Autodesk Inventor part; units mm, degrees
ref_plane "YZ Plane" through (0, 0, 0) normal (1, 0, 0) x (0, 1, 0)
ref_plane "XZ Plane" through (0, 0, 0) normal (0, 1, 0) x (-1, 0, 0)
ref_plane "XY Plane" through (0, 0, 0) normal (0, 0, 1) x (1, 0, 0)
sketch "スケッチ1" plane through (0, 0, 0) normal (0, 1, 0) x (-1, 0, 0)
  circle A0 centre (0, 0) radius 1.15
  circle A1 centre (0, 0) radius 2
  circle A2 centre (0, 0) radius 5
  line L0 (0, 0) -> (7, 0)
  line L1 (7, 0) -> (7, 4.5)
  line L2 (7, 4.5) -> (0, 4.5)
  line L3 (0, 4.5) -> (0, 0)
  line L4 (0, 0) -> (7, 0)
  line L5 (7, 0) -> (7, -5)
  line L6 (7, -5) -> (0, -5)
  line L7 (0, -5) -> (0, 0)
  line L8 (0, 4.5) -> (-2, 4.5)
  line L9 (-2, 4.5) -> (-2, 0)
  line L10 (-2, 0) -> (0, 0)
  line L11 (0, 0) -> (0, 4.5)
  circle A3 centre (0, 0) radius 3
  line L12 (-2, 0) -> (-2, -5)
  line L13 (-2, -5) -> (0, -5)
  line L14 (2, 0) -> (2, -5)
  circle A4 centre (0, 0) radius 4.9244
  line L15 (-2, 0) -> (-4.9244, 0)
  line L16 (0, -4.9244) -> (0, -5.9244)
  line L17 (0, -5.9244) -> (7, -5.9244)
  line L18 (7, -5.9244) -> (7, -5)
  line L19 (7, -5) -> (0, -5.9244)
  line L20 (0, -5.9244) -> (4.9138, -5)
  line L21 (0, -5) -> (0, -7)
  line L22 (0, -7) -> (4.9138, -5)
  point P0 (0, 2)
  point P1 (-2, 2.2361)
  point P2 (-2, -2.2361)
  point P3 (-2, -4.5826)
  point P4 (-2, -4.5)
  point P5 (0, -4.9244)
  dimension "d2" = 10
  dimension "d0" = 2.3
  dimension "d1" = 4
  dimension "d3" = 7
  dimension "d4" = 4.5
  dimension "d5" = 6
  dimension "d22" = 1
  dimension "d34" = 5
  dimension "d39" = 2
extrude "押し出し1" add sketch "スケッチ1" along normal blind 4.5 contours A1 L3 A3 L0 | L0 A3 L14 | A3 L3 L2 A4 L0 | L0 A4 L14 A3 | A4 L2 A2 L0 | L0 A2 L14 A4 | L0 L5 L6 L14 A2 | A2 L2 L1 L0
extrude "押し出し2" add sketch "スケッチ1" along normal blind 3 contours A1 L9 A3 L3 | L15 A3 L9 | L12 A3 L15 | A3 L9 L8 L3 | A3 L15 A4 L9 | L12 A4 L15 A3
extrude "押し出し3" add sketch "スケッチ1" against normal blind 1 contours L0 A1 L7 A0 | A0 L3 A1 L0 | A0 L10 A1 L3 | L7 A1 L10 A0 | L14 A3 L7 A1 | A1 L3 A3 L0 | L0 A3 L14 | A1 L9 A3 L3 | L7 A3 L12 A1 | A3 L3 L2 A4 L0 | L0 A4 L14 A3 | L14 A4 L7 A3 | L15 A3 L9 | L12 A3 L15 | A3 L9 L8 L3 | L7 A4 L12 A3 | A4 L2 A2 L0 | L0 A2 L14 A4 | L14 A2 L7 A4 | A3 L15 A4 L9 | L12 A4 L15 A3 | L0 L5 L6 L14 A2 | A2 L2 L1 L0 | L14 L6 A2 | L6 L20 L16 | L19 L22 L17 | L20 L22 L19 | L17 L22 L21
sketch "スケッチ2" plane through (0, 4.5, 0) normal (0, 1, 0) x (1, 0, 0)
  circle A0 centre (0, 0) radius 1.15
  circle A1 centre (0, 0) radius 2
  circle A2 centre (0, 0) radius 4.9244
  line L0 (0, 0) -> (2, 0)
  line L1 (2, 0) -> (2, -4.5)
  line L2 (2, -4.5) -> (0, -4.5)
  line L3 (0, -4.5) -> (0, 0)
  line L4 (-2, 5) -> (-7, 5)
  line L5 (0, -4.5) -> (-7, -4.5)
  line L6 (-7, -4.5) -> (-7, 5)
  line L7 (-7, 5) -> (0, 5)
  line L8 (0, 5) -> (0, -4.5)
  line L9 (0, 0) -> (2, 0)
  line L10 (2, 0) -> (2, 5)
  line L11 (2, 5) -> (0, 5)
  line L12 (0, 5) -> (0, 0)
  line L13 (0, 5) -> (-7, 5)
  line L14 (0, 5.9244) -> (0, 5)
  line L15 (-7, 5) -> (0, 5.9244)
  line L16 (0, 5.9244) -> (-4.9138, 5)
  line L17 (-2, 5) -> (-7, 5)
  line L18 (0, 5) -> (0, 7)
  line L19 (0, 7) -> (-4.9138, 5)
  point P0 (0, 4.9244)
  dimension "d12" = 4
  dimension "d35" = 5
  dimension "d40" = 2
extrude "押し出し4" add sketch "スケッチ2" along normal blind 1 contours L0 A1 L3 A0 | A0 L8 A1 L0 | A0 L3 A1 L8 | L1 L2 L3 A1 | L10 A2 L1 | A1 L8 A2 L10 | A1 L3 L5 A2 L8 | A2 L5 L6 L4 L7 L8 | L7 L4 L16 L14 | L16 L19 L15 | L15 L19 L18
sketch "スケッチ4" plane through (0, 3, 4.5) normal (0, 0, 1) x (1, 0, 0)
  line L0 (-7, 2.5) -> (2, 2.5)
  line L1 (-7, 2.5) -> (-4.5, 2.5)
  line L2 (-4.5, 2.5) -> (-4.5, -0.75)
  line L3 (-4.5, -0.75) -> (-7, -0.75)
  line L4 (-7, -0.75) -> (-7, 2.5)
  circle A0 centre (-4.5, -0.75) radius 1.4
  line L5 (0, -3) -> (0, -2.5)
  line L6 (0, -2.5) -> (-1.5, -2.5)
  circle A1 centre (-1.5, -2.5) radius 0.5
  dimension "d23" = 2.5
  dimension "d24" = 3.25
  dimension "d25" = 2.8
  dimension "d26" = 0.5
  dimension "d27" = 1.5
  dimension "d28" = 1
extrude "押し出し6" cut sketch "スケッチ4" against normal blind 6 contours A0 L3 L2 | L2 L3 A0 | A1
chamfer "面取り2" distance 2 angle 45 3 edges at (-7, 5.5, -0.25) (-7, -1, -0.25) (-7, 2.25, -5)
properties part number "rod5.6"
Part model, mm, in its own coordinate system. A direction names the side the tool comes from. Give positions to 0.01 mm unless a question says otherwise; leave off trailing zeros. Loops run counter-clockwise (first coordinate to the right, second up) from the corner with the lowest first, then second, coordinate; pieces in that order, holes last. Notation, with made-up numbers: M -36,-39 L -24,-39 A21 ccw -24,-2 Z; hole C -37,13.25 d11. An arc over 180 degrees is marked long. Put each result on its own line as item: value. Start each with the question number.
1) 3-axis set-ups, long thin cutter, end or side, ignore diameter. For faces 1 (the flat face through (-2, 2, -2)), 2 (the flat face through (-5, 2, -1.5)), 3 (the flat face through (0, 5, -6)): which of +Z, -Z, +X, -X, +Y, -Y reach the whole face in a straight line?
2) Saw through at B-B (z = -6). List the corners of the cut face in (x, y).
3) Saw through at C-C (y = 2.75). List the corners of the cut face in (x, z).
4) Saw through at A-A (x = -0.75). List the corners of the cut face in (y, z).
5) Probe probe 1 along Y at (x, z) = (1, -2.75); probe 2 along Y at (x, z) = (1.5, 2.5); probe 3 along X at (y, z) = (2.75, 1). List the from-to ranges inside material, lowest first.
6) Flat gauge pins, fed straight in: pin 1 (2 mm diameter, centred on y = 2, z = -3, fed in from +X); pin 2 (2.5 mm diameter, centred on x = 0, z = 0, fed in from +Y); pin 3 (1.5 mm diameter, centred on y = 0, z = 1, fed in from +X); pin 4 (2.5 mm diameter, centred on x = -3, y = 3, fed in from -Z). Where does each tip first touch, or does it go through?
7) Saw through at D-D (x = 3.25). List the corners of the cut face in (y, z), then the cut area to 3 significant figures.
8) Pull direction Y, two halves, no side cores. Call faces 4 (the cylindrical face through (0.91, -0.49, -0.7)), 5 (the flat face through (-1, -1, -1)), 6 (the flat face through (0, 4, 3)): +Y half, -Y half, draft (parallel to the pull), parting line (faces both ways), or undercut.
Numbers:
1. face 1: -Z
1. face 2: +Z
1. face 3: -Z, +X, +Y, -Y
2. outline: M -2.46,-1 L 0,-1 L 0,0 L -2.46,0 Z; M -2.46,4.5 L 0,4.5 L 0,5.5 L -2.46,5.5 Z
3. outline: M -7,-3 L -5,-5 L -2,-5 L -2,0 A2 cw 2,0 L 2,-4.5 A4.92 ccw 2,4.5 L -3.19,4.5 L -3.19,-1.5 L -5.81,-1.5 L -5.81,4.5 L -7,4.5 Z
4. outline: M -1,-6.69 L 0,-6.69 L 0,-0.87 L -1,-0.87 Z; M -1,0.87 L 0,0.87 L 0,1.85 L 4.5,1.85 L 4.5,0.87 L 5.5,0.87 L 5.5,4.5 L -1,4.5 Z; M 4.5,-6.69 L 5.5,-6.69 L 5.5,-0.87 L 4.5,-0.87 Z
5. probe 1: -1 to 0, 4.5 to 5.5
5. probe 2: -1 to 3, 4.5 to 5.5
5. probe 3: -7 to -5.81, -3.19 to -1.73, 1.73 to 4.82
6. pin 1: x = 4.5
6. pin 2: y = 5.5
6. pin 3: x = 4.92
6. pin 4: z = -5
7. outline: M -1,-3.7 L 3,-3.7 L 3,3.7 L -1,3.7 Z; M 4.5,-3.7 L 5.5,-3.7 L 5.5,3.7 L 4.5,3.7 Z
7. area: 37.0 mm^2
8. face 4: draft
8. face 5: -Y half
8. face 6: undercut
